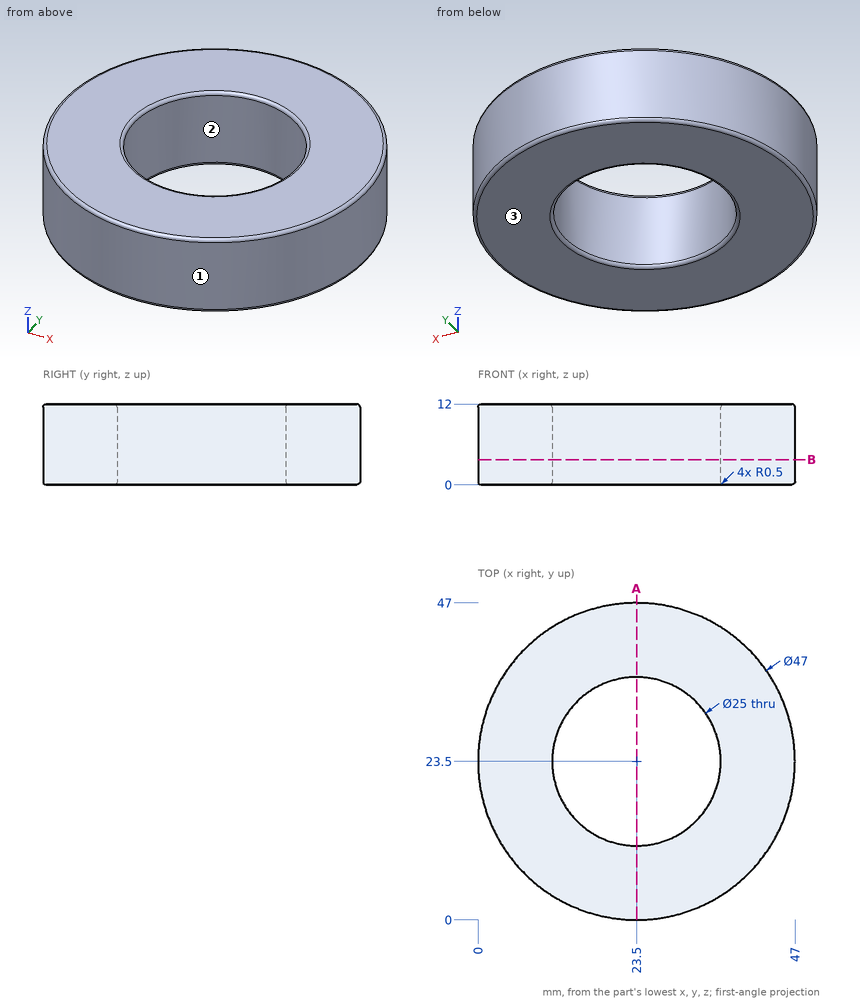
Here's the drawing with two shaded views (mm, measured from the low corner). I have some questions. Give positions to 0.01 mm unless a question says otherwise; leave off trailing zeros. Order: outer loops, then holes, each group sorted by start corner. A loop starts at its lowest first (then second) coordinate and runs counter-clockwise, first axis right, second up. Notation, with made-up numbers: M 51,54.25 L 97,54.25 A27 cw 97,70.25 Z; hole C 32.5,7 d7. An arc over 180 degrees is marked long. Answer as a JSON object with one key per item and string values. Group by question number.
1) We'd pull the mould along Y, two halves only. Please class the marked faces 1, 2 and 3: pulls with the +Y half, pulls with the -Y half, needs draft (parallel to the pull), parting line crosses it, or undercut.
2) Please list where these lines run through material, in increasing order: L1, parallel to Y at x = 23.5, z = 4.75; L2, parallel to Y at x = 16.5, z = 10.75; L3, parallel to X at y = 34, z = 10.75. Write a range as [from, to].
3) Suppose I cut it at A-A, the plane x = 23.5. Write out the boundary of the cut face in (y, z).
4) Suppose I cut it at B-B, the plane z = 3.75. Write out the boundary of the cut face in (x, y), plus the area to 3 significant figures.
5) I'm going to push flat-ended pins straight in: pin 1 Ø1.5 at (y, z) = (5, 9.5) entering from +X; pin 2 Ø1 at (y, z) = (38, 1.5) entering from -X; pin 3 Ø6 at (x, z) = (34, 9.5) entering from +Y. Where does each tip first touch, or does it pass through?
Results found:
{
 "1": {"face 1": "parting line crosses it", "face 2": "undercut", "face 3": "needs draft"},
 "2": {"L1": "[0, 11], [36, 47]", "L2": "[1.07, 13.14], [33.86, 45.93]", "L3": "[2.48, 16.72], [30.28, 44.52]"},
 "3": {"outline": "M 0,0.5 A0.5 ccw 0.5,0 L 10.5,0 A0.5 ccw 11,0.5 L 11,11.5 A0.5 ccw 10.5,12 L 0.5,12 A0.5 ccw 0,11.5 Z; M 36,0.5 A0.5 ccw 36.5,0 L 46.5,0 A0.5 ccw 47,0.5 L 47,11.5 A0.5 ccw 46.5,12 L 36.5,12 A0.5 ccw 36,11.5 Z"},
 "4": {"outline": "C 23.5,23.5 d47; hole C 23.5,23.5 d25", "area": "1,240 mm²"},
 "5": {"pin 1": "x = 38.9", "pin 2": "x = 4.63", "pin 3": "y = 45.77"}
}
